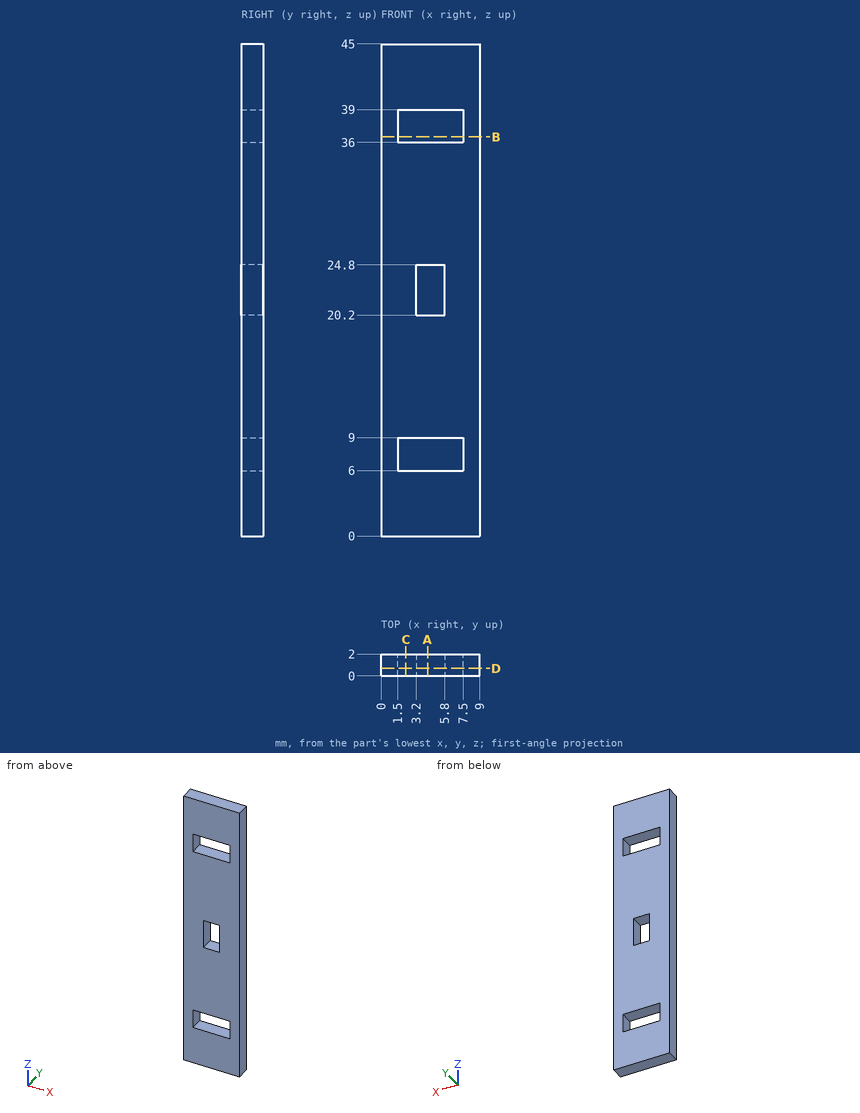
Here's the drawing with two shaded views (mm, measured from the low corner). I have some questions. Give positions to 0.01 mm unless a question says otherwise; leave off trailing zeros. Loops run counter-clockwise (first coordinate to the right, second up) from the corner with the lowest first, then second, coordinate; pieces in that order, holes last. Notation, with made-up numbers: M -4,-31.75 L 34,-31.75 A33 cw 34,4.25 Z; hole C -6,-16.75 d10. An arc over 180 degrees is marked long. Answer in a Markdown table with one row per item.
1. Suppose I cut it at D-D on y = 0.7. Write out the boundary of the cut face in (x, z), plus the area to 3 significant figures.
Taken from the geometry:
| item | result |
|---|---|
| outline | M 0,0 L 9,0 L 9,45 L 0,45 Z; hole M 1.5,6 L 7.5,6 L 7.5,9 L 1.5,9 Z; hole M 1.5,36 L 7.5,36 L 7.5,39 L 1.5,39 Z; hole M 3.2,20.2 L 5.8,20.2 L 5.8,24.8 L 3.2,24.8 Z |
| area | 357 mm² |
2. Suppose I cut it at A-A on x = 4.25. Write out the boundary of the cut face in (y, z).
Taken from the geometry:
| item | result |
|---|---|
| outline | M 0,0 L 2,0 L 2,6 L 0,6 Z; M 0,9 L 2,9 L 2,20.2 L 0,20.2 Z; M 0,24.8 L 2,24.8 L 2,36 L 0,36 Z; M 0,39 L 2,39 L 2,45 L 0,45 Z |
3. Suppose I cut it at B-B on z = 36.5. Write out the boundary of the cut face in (x, y).
Taken from the geometry:
| item | result |
|---|---|
| outline | M 0,0 L 1.5,0 L 1.5,2 L 0,2 Z; M 7.5,0 L 9,0 L 9,2 L 7.5,2 Z |
4. Suppose I cut it at C-C on x = 2.25. Write out the boundary of the cut face in (y, z), plus the area to 3 significant figures.
Taken from the geometry:
| item | result |
|---|---|
| outline | M 0,0 L 2,0 L 2,6 L 0,6 Z; M 0,9 L 2,9 L 2,36 L 0,36 Z; M 0,39 L 2,39 L 2,45 L 0,45 Z |
| area | 78.0 mm² |
5. If I drill on line 1 along Z through (x, y) = (6.25, 0.7); line 2 along Z through (x, y) = (4.75, 1.95); line 3 along X through (y, z) = (1.4, 6.5), over which ranges is the centre line in solid material (lowest first)?
Taken from the geometry:
| item | result |
|---|---|
| line 1 | z = 0 to 6, 9 to 36, 39 to 45 |
| line 2 | z = 0 to 6, 9 to 20.2, 24.8 to 36, 39 to 45 |
| line 3 | x = 0 to 1.5, 7.5 to 9 |
